from build123d import *

# Parameters (mm, degrees)
MODEL_R             = 2.7
MODEL_R_2           = 3.875
MODEL_R_3           = 12
MODEL_R_4           = 1.6
BOSS_EXTRUDE1_DEPTH = 3.125
FILLET1_R           = 10


with BuildPart() as part:
    # Model → Boss-Extrude1 (new body)
    with BuildSketch(Plane.XY):
        Polygon((-0.063524835, 46), (-0.063524835, 20), (60, 0), (122.936475165, 0), (122.936475165, 66), (59.936475165, 66), align=None)
        with Locations((69.936475165, 8)):
            Circle(MODEL_R, mode=Mode.SUBTRACT)
        with Locations((9.936475165, 33)):
            Circle(MODEL_R_2, mode=Mode.SUBTRACT)
        with Locations((69.936475165, 58)):
            Circle(MODEL_R, mode=Mode.SUBTRACT)
        with Locations((102.436475165, 33)):
            Circle(MODEL_R_3, mode=Mode.SUBTRACT)
        with Locations((86.936475165, 48.5)):
            Circle(MODEL_R_4, mode=Mode.SUBTRACT)
        with Locations((117.936475165, 48.5)):
            Circle(MODEL_R_4, mode=Mode.SUBTRACT)
        with Locations((86.936475165, 17.5)):
            Circle(MODEL_R_4, mode=Mode.SUBTRACT)
        with Locations((117.936475165, 17.5)):
            Circle(MODEL_R_4, mode=Mode.SUBTRACT)
    extrude(amount=BOSS_EXTRUDE1_DEPTH)

    # Fillet1
    fillet1_edges = [part.edges().sort_by_distance(p)[0] for p in [
        (59.936475165, 66, 1.5625),
        (122.936475165, 66, 1.5625),
        (122.936475165, 0, 1.5625),
        (60, 0, 1.5625),
        (-0.063524835, 20, 1.5625),
        (-0.063524835, 46, 1.5625),
    ]]
    fillet(fillet1_edges, radius=FILLET1_R)


solid = part.part
Verification items for the finished model (mm, model axes). Give positions to 0.01 mm unless a question says otherwise; leave off trailing zeros. Loops run counter-clockwise (first coordinate to the right, second up) from the corner with the lowest first, then second, coordinate; pieces in that order, holes last.
1. Release check for a two-part mould opening along X. For faces 1 (the flat face through (87, 0, 2)), 2 (the cylindrical face through (9.096, 29.217, 1.541)), 3 (the cylindrical face through (119.93, 63.15, 1.58)) record: +X half, -X half, draft (parallel to the pull), parting line (faces both ways), or undercut.
Derived:
face 1: draft
face 2: undercut
face 3: +X half
2. Cross-section at B-B on y = 8. Record the cut outline in (x, z) (3 decimals), and give its area (3 significant figures).
Derived:
outline: (35.975, 0) - (67.236, 0) - (67.236, 3.125) - (35.975, 3.125) - close; (72.636, 0) - (122.734, 0) - (122.734, 3.125) - (72.636, 3.125) - close
area: 254 mm2
3. Cross-section at D-D on x = 39. Record the cut outline in (y, z) (3 decimals).
Derived:
outline: (6.993, 0) - (59.021, 0) - (59.021, 3.125) - (6.993, 3.125) - close
4. Material ranges on probe 1 along Y at (x, z) = (102, 1.4); probe 2 along Y at (x, z) = (113, 1.3); probe 3 along X at (y, z) = (24, 1.4), recorded low to high.
Derived:
probe 1: y = 0 to 21.01, 44.99 to 66
probe 2: y = 0 to 27.31, 38.69 to 66
probe 3: x = 0.47 to 94.5, 110.37 to 122.94
5. Cross-section at C-C on x = 12. Record the cut outline in (y, z) (3 decimals).
Derived:
outline: (15.983, 0) - (29.72, 0) - (29.72, 3.125) - (15.983, 3.125) - close; (36.28, 0) - (50.021, 0) - (50.021, 3.125) - (36.28, 3.125) - close
6. Go/stop test with flat-tipped pins: P1, Ø3, axis at x = 117.94, y = 17.5, coming from the +Z side; P2, Ø1.5, axis at x = 41, z = 2, coming from the +Y side. Record where each tip stops, or that it passes through.
Derived:
P1: passes through
P2: stops at y = 59.94
7. Cross-section at A-A on z = 1.1. Count the separate pieces of the cut face and the enclosed holes in it, and give its area (3 significant figures).
Derived:
separate pieces: 1
enclosed holes: 8
area: 6,280 mm2
